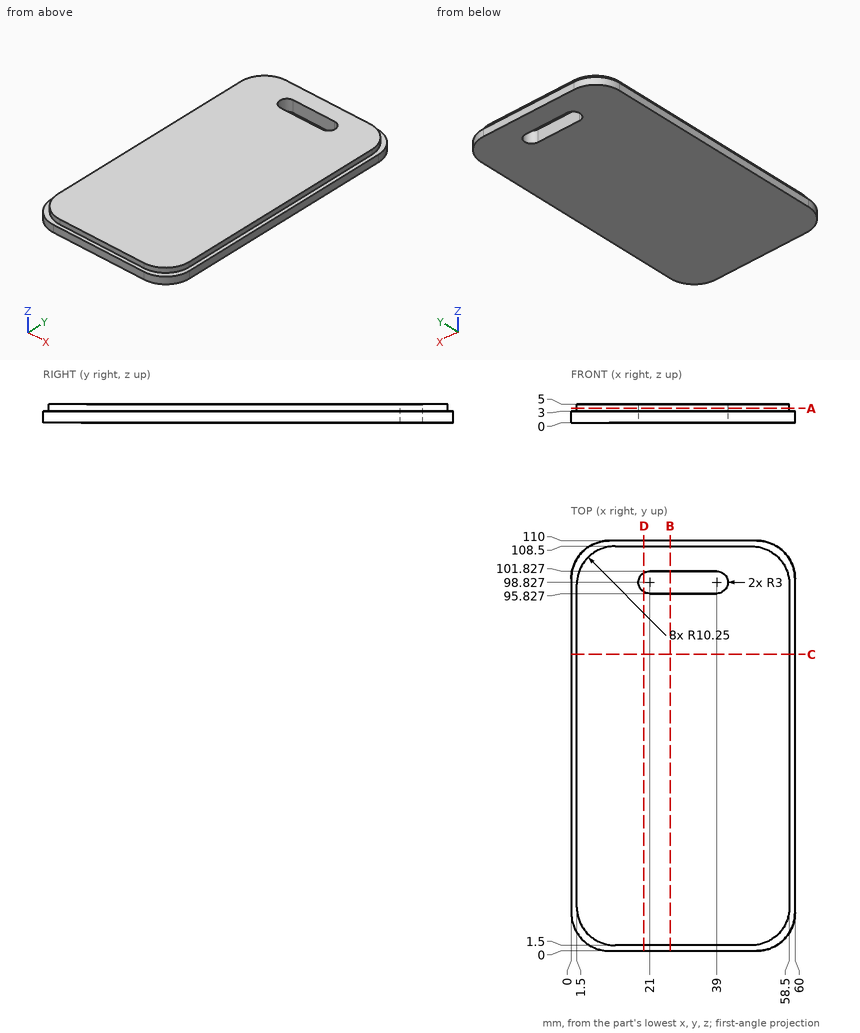
Input: dimensioned drawing with shaded views. Units: mm. Origin: part minimum x, y, z. Give positions to 0.01 mm unless a question says otherwise; leave off trailing zeros. Write each loop counter-clockwise with the first axis right and the second up, starting at its lowest first coordinate (ties: lowest second). Pieces come first, ordered by that corner, then holes.
1. Section query B-B (x = 26.5). Return the cut outline in (y, z), then the cut area to 3 significant figures.
2. Material intervals for line 1 along Y through (x, z) = (29, 1.8); line 2 along Y through (x, z) = (14, 4.6); line 3 along X through (y, z) = (69, 4), sorted ascending.
3. Section query A-A (z = 3.85). Return the cut outline in (x, y), then the cut area to 3 significant figures.
4. First-contact query: pin 1 (1 mm diameter, centred on x = 45.5, z = 4.5, fed in from +Y); pin 2 (0.6 mm diameter, centred on x = 26.5, z = 4, fed in from -Y); pin 3 (0.6 mm diameter, centred on y = 63.5, z = 4, fed in from -X). Flat tips, straight axial feed; report the tip coordinate or a pass-through.
5. Section query D-D (x = 19.5). Return the cut outline in (y, z) (1 decimal).
6. Section query C-C (y = 79.5). Return the cut outline in (x, z).
Output values:
1. outline: (0, 0) - (95.83, 0) - (95.83, 5) - (1.5, 5) - (1.5, 3) - (0, 3) - close; (101.83, 0) - (110, 0) - (110, 3) - (108.5, 3) - (108.5, 5) - (101.83, 5) - close
1. area: 514 mm2
2. line 1: y = 0 to 95.83, 101.83 to 110
2. line 2: y = 1.5 to 108.5
2. line 3: x = 1.5 to 58.5
3. outline: (1.5, 11.75) arc R10.25 ccw to (11.75, 1.5) - (48.25, 1.5) arc R10.25 ccw to (58.5, 11.75) - (58.5, 98.25) arc R10.25 ccw to (48.25, 108.5) - (11.75, 108.5) arc R10.25 ccw to (1.5, 98.25) - close; hole (21, 95.83) - (39, 95.83) arc R3 ccw to (39, 101.83) - (21, 101.83) arc R3 ccw to start
3. area: 5,870 mm2
4. pin 1: stops at y = 108.5
4. pin 2: stops at y = 1.5
4. pin 3: stops at x = 1.5
5. outline: (0, 0) - (96.2, 0) - (96.2, 5) - (1.5, 5) - (1.5, 3) - (0, 3) - close; (101.4, 0) - (110, 0) - (110, 3) - (108.5, 3) - (108.5, 5) - (101.4, 5) - close
6. outline: (0, 0) - (60, 0) - (60, 3) - (58.5, 3) - (58.5, 5) - (1.5, 5) - (1.5, 3) - (0, 3) - close
